The listing builds one solid part. Answer for the finished solid, in the listing's coordinates (mm). A direction names the side the tool comes from. Give positions to 0.01 mm unless a question says otherwise; leave off trailing zeros. Write each loop counter-clockwise with the first axis right and the second up, starting at its lowest first coordinate (ties: lowest second). Pieces come first, ordered by that corner, then holes. Notation, with made-up numbers: (8.5, 78) - (40.5, 78) arc R32 cw to (40.5, 115) - close; hole circle Ø6 at (24, 57.25). An arc over 180 degrees is marked (long way). Return JSON: item names as keys, results as strings.
from build123d import *

# Parameters (mm, degrees)
F0_R     = 2.5
F1_DEPTH = 8.6
F2_R     = 2.5
F3_R     = 2.95
F4_DEPTH = 1


with BuildPart() as f1:
    # F0 (on Top) → F1 (new body)
    with BuildSketch(Plane.XY):
        Circle(F0_R)
    extrude(amount=F1_DEPTH)

    # F2
    f2_edges = [f1.edges().sort_by_distance(p)[0] for p in [
        (-2.5, 0, 8.6),
    ]]
    fillet(f2_edges, radius=F2_R)

    # F3 (on face) → F4 (join)
    with BuildSketch(Plane(origin=(0, 0, 0), x_dir=(1, 0, 0), z_dir=(0, 0, -1))):
        Circle(F3_R)
    extrude(amount=-F4_DEPTH)


solid = f1.part
Item 1: For faces 1 (the face through (0, 0, 0)), 2 (the face through (-0.54, -2.44, 3.51)), determine the directions among +Z, -Z, +X, -X, +Y, -Y from which every point of the face is accessible in a straight line to the end or side of a thin tool.
Answer below:
{"face 1": "-Z, +X, -X, +Y, -Y", "face 2": "+Z"}
Item 2: A cutting plane is placed at C-C on z = 3.25. Determine the outline of the cut face in (x, y), then the cut area to 3 significant figures.
Answer below:
{"outline": "circle Ø5 at (0, 0)", "area": "19.6 mm²"}
Item 3: Flat-ended cylindrical pins translate along their axes: P1, Ø2, axis at x = 2, z = 5.5, coming from the -Y side; P2, Ø2, axis at x = 1.5, z = 3.5, coming from the -Y side. Find the tip coordinate at first contact, or state that the pin passes through.
Answer below:
{"P1": "stops at y = -2.29", "P2": "stops at y = -2.45"}
Item 4: Consider L1, parallel to Z at x = -2.5, y = 1.1; L2, parallel to X at y = 0, z = 4; L3, parallel to Y at x = 0.35, z = 3. Determine where each line is inside the solid, lowest interval first.
Answer below:
{"L1": "z = 0 to 1", "L2": "x = -2.5 to 2.5", "L3": "y = -2.48 to 2.48"}
Item 5: A cutting plane is placed at A-A on x = 0. Determine the outline of the cut face in (y, z), then the cut area to 3 significant figures.
Answer below:
{"outline": "(-2.95, 0) - (2.95, 0) - (2.95, 1) - (2.5, 1) - (2.5, 6.1) arc R2.5 ccw to (-2.5, 6.1) - (-2.5, 1) - (-2.95, 1) - close", "area": "41.2 mm²"}
